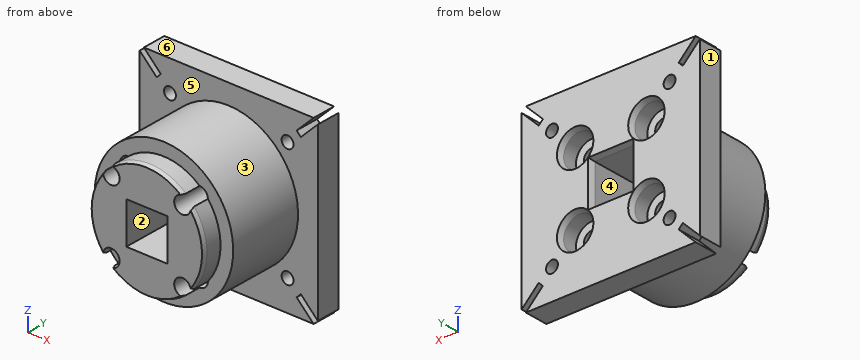
from build123d import *

# Parameters (mm, degrees)
SKETCH1_R           = 17.5
BOSS_EXTRUDE1_DEPTH = 25
SKETCH3_R           = 14.3
BOSS_EXTRUDE2_DEPTH = 5
SKETCH4_W           = 10.4
SKETCH4_H           = 10.4
CUT_EXTRUDE1_DEPTH  = 39.890872965
SKETCH6_R           = 2.1
CUT_EXTRUDE2_DEPTH  = 39.890872965
CHAMFER1_SIZE       = 0.363970234
CHAMFER1_SIZE_2     = 1
SKETCH7_R           = 4.1
CUT_EXTRUDE3_DEPTH  = 5
CHAMFER2_SIZE       = 0.5
CHAMFER2_SIZE2      = 1.37373871
BOSS_EXTRUDE3_START = -6
SKETCH8_W           = 45
SKETCH8_H           = 45
SKETCH8_R           = 17.5
SKETCH8_R_2         = 1.5
BOSS_EXTRUDE3_DEPTH = 6
CUT_EXTRUDE4_DEPTH  = 44.73213928
CHAMFER3_SIZE       = 0.5
CHAMFER3_SIZE2      = 1.37373871


with BuildPart() as part:
    # Sketch1 → Boss-Extrude1 (new body)
    with BuildSketch(Plane(origin=(0, 0, 0), x_dir=(1, 0, 0), z_dir=(0, 1, 0))):
        with Locations(Location((0, 0, 0), (0, 0, 270))):
            Circle(SKETCH1_R)
    extrude(amount=BOSS_EXTRUDE1_DEPTH)

    # Sketch3 → Boss-Extrude2 (add)
    with BuildSketch(Plane.XZ):
        with Locations(Location((0, 0, 0), (0, 0, 90))):
            Circle(SKETCH3_R)
    extrude(amount=BOSS_EXTRUDE2_DEPTH)

    # Sketch4 → Cut-Extrude1 (cut, through all)
    with BuildSketch(Plane(origin=(0, 25, 0), x_dir=(1, 0, 0), z_dir=(0, 1, 0))):
        Rectangle(SKETCH4_W, SKETCH4_H)
    extrude(amount=-CUT_EXTRUDE1_DEPTH, mode=Mode.SUBTRACT)

    # Sketch6 → Cut-Extrude2 (cut, through all)
    with BuildSketch(Plane(origin=(0, 25, 0), x_dir=(1, 0, 0), z_dir=(0, 1, 0))):
        with Locations(Location((9, -9, 0), (0, 0, 270))):
            Circle(SKETCH6_R)
        with Locations(Location((-9, -9, 0), (0, 0, 270))):
            Circle(SKETCH6_R)
        with Locations(Location((-9, 9, 0), (0, 0, 270))):
            Circle(SKETCH6_R)
        with Locations(Location((9, 9, 0), (0, 0, 270))):
            Circle(SKETCH6_R)
    extrude(amount=-CUT_EXTRUDE2_DEPTH, mode=Mode.SUBTRACT)

    # Chamfer1
    # the kernel refuses this chamfer: 1, 0.363970234 mm, written as the material it takes off along each edge
    with BuildSketch(Plane(origin=(0, -5, 0), x_dir=(-0.7601968687413804, 0, 0.649692789521171), z_dir=(-0.649692789521171, 0, -0.7601968687413804))) as chamfer1_piece_1:
        Polygon((14.3 - CHAMFER1_SIZE, 0), (14.3, CHAMFER1_SIZE_2), (14.3, 0), align=None)
    revolve(axis=Axis((0, -5, 0), (0, 1, 0)), revolution_arc=98.963112953, mode=Mode.SUBTRACT)
    with BuildSketch(Plane(origin=(0, -5, 0), x_dir=(-0.6496927895211715, 0, 0.7601968687413799), z_dir=(0.7601968687413799, 0, 0.6496927895211715))) as chamfer1_piece_2:
        Polygon((14.3 - CHAMFER1_SIZE, 0), (14.3, -CHAMFER1_SIZE_2), (14.3, 0), align=None)
    revolve(axis=Axis((0, -5, 0), (0, -1, 0)), revolution_arc=98.963112953, mode=Mode.SUBTRACT)
    with BuildSketch(Plane(origin=(0, -5, 0), x_dir=(-0.7601968687413795, 0, -0.6496927895211719), z_dir=(-0.6496927895211719, 0, 0.7601968687413795))) as chamfer1_piece_3:
        Polygon((14.3, -CHAMFER1_SIZE_2), (14.3 - CHAMFER1_SIZE, 0), (14.3, 0), align=None)
    revolve(axis=Axis((0, -5, 0), (0, -1, 0)), revolution_arc=98.963112953, mode=Mode.SUBTRACT)
    with BuildSketch(Plane(origin=(0, -5, 0), x_dir=(0.6496927895211716, 0, -0.7601968687413798), z_dir=(-0.7601968687413798, 0, -0.6496927895211716))) as chamfer1_piece_4:
        Polygon((14.3, -CHAMFER1_SIZE_2), (14.3 - CHAMFER1_SIZE, 0), (14.3, 0), align=None)
    revolve(axis=Axis((0, -5, 0), (0, -1, 0)), revolution_arc=98.963112953, mode=Mode.SUBTRACT)

    # Sketch7 → Cut-Extrude3 (cut)
    with BuildSketch(Plane(origin=(0, 25, 0), x_dir=(1, 0, 0), z_dir=(0, 1, 0))):
        with Locations(Location((9, 9, 0), (0, 0, 270))):
            Circle(SKETCH7_R)
        with Locations(Location((-9, 9, 0), (0, 0, 270))):
            Circle(SKETCH7_R)
        with Locations(Location((-9, -9, 0), (0, 0, 270))):
            Circle(SKETCH7_R)
        with Locations(Location((9, -9, 0), (0, 0, 270))):
            Circle(SKETCH7_R)
    extrude(amount=-CUT_EXTRUDE3_DEPTH, mode=Mode.SUBTRACT)

    # Chamfer2
    chamfer2_edges = [part.edges().sort_by_distance(p)[0] for p in [
        (5.2, 25, 0),
        (0, 25, -5.2),
        (-5.2, 25, 0),
        (0, 25, 5.2),
    ]]
    chamfer2_side = [part.faces().sort_by_distance(p)[0] for p in [
        (0, 25, -17.005025253),
    ]]
    chamfer(chamfer2_edges, length=CHAMFER2_SIZE, length2=CHAMFER2_SIZE2, reference=chamfer2_side[0])

    # Sketch8 → Boss-Extrude3 (add)
    with BuildSketch(Plane(origin=(0, 25, 0), x_dir=(1, 0, 0), z_dir=(0, 1, 0)).offset(BOSS_EXTRUDE3_START)):
        Rectangle(SKETCH8_W, SKETCH8_H)
        with Locations(Location((0, 0, 0), (0, 0, 270))):
            Circle(SKETCH8_R, mode=Mode.SUBTRACT)
        with Locations(Location((-14.849242405, -14.849242405, 0), (0, 0, 270))):
            Circle(SKETCH8_R_2, mode=Mode.SUBTRACT)
        with Locations(Location((-14.849242405, 14.849242405, 0), (0, 0, 270))):
            Circle(SKETCH8_R_2, mode=Mode.SUBTRACT)
        with Locations(Location((14.849242405, 14.849242405, 0), (0, 0, 270))):
            Circle(SKETCH8_R_2, mode=Mode.SUBTRACT)
        with Locations(Location((14.849242405, -14.849242405, 0), (0, 0, 270))):
            Circle(SKETCH8_R_2, mode=Mode.SUBTRACT)
    extrude(amount=BOSS_EXTRUDE3_DEPTH)

    # Sketch10 → Cut-Extrude4 (cut, through all)
    with BuildSketch(Plane(origin=(0, 25, 0), x_dir=(1, 0, 0), z_dir=(0, 1, 0))):
        Polygon((-18.207999616, -17.147339444), (-17.147339444, -18.207999616), (-21.439339828, -22.5), (-22.5, -22.5), (-22.5, -21.439339828), align=None)
        Polygon((-22.5, 21.439339828), (-18.207999616, 17.147339444), (-17.147339444, 18.207999616), (-21.439339828, 22.5), (-22.5, 22.5), align=None)
        Polygon((21.439339828, 22.5), (17.147339444, 18.207999616), (18.207999616, 17.147339444), (22.5, 21.439339828), (22.5, 22.5), align=None)
        Polygon((17.147339444, -18.207999616), (18.207999616, -17.147339444), (22.5, -21.439339828), (22.5, -22.5), (21.439339828, -22.5), align=None)
    extrude(amount=-CUT_EXTRUDE4_DEPTH, mode=Mode.SUBTRACT)

    # Chamfer3
    chamfer3_edges = [part.edges().sort_by_distance(p)[0] for p in [
        (-9, 25, -13.1),
        (-9, 25, 4.9),
        (9, 25, 4.9),
        (9, 25, -13.1),
    ]]
    chamfer3_side = [part.faces().sort_by_distance(p)[0] for p in [
        (18.843339636, 25, -20.803999808),
    ]]
    chamfer(chamfer3_edges, length=CHAMFER3_SIZE, length2=CHAMFER3_SIZE2, reference=chamfer3_side[0])


solid = part.part
Input: part model. Units: mm. Frame: model coordinates. Face numbers are marked on the shaded views. A direction names the side the tool comes from. Give positions to 0.01 mm unless a question says otherwise; leave off trailing zeros. Order: outer loops, then holes, each group sorted by start corner. A loop starts at its lowest first (then second) coordinate and runs counter-clockwise, first axis right, second up. Notation, with made-up numbers: (-38, -30.75) - (14, -30.75) arc R29 ccw to (14, 0.25) - close; hole circle Ø9 at (18.5, 57.25). An arc over 180 degrees is marked (long way). Write each question's results on one line, items separated by ' | '.
Item 1: Access query for the marked faces 1, 2 and 3. Directions: +Z, -Z, +X, -X, +Y, -Y. A direction counts if a zero-diameter tool reaches every point of the face in a straight line with its end or side. Return the directions, or none.
A:
face 1: +Z, -Z, -X, +Y, -Y | face 2: +Y, -Y | face 3: -Y
Item 2: Material intervals for line 1 along X through (y, z) = (1.5, 0); line 2 along X through (y, z) = (19.5, -2); line 3 along X through (y, z) = (21, -9), sorted ascending.
A:
line 1: x = -17.5 to -5.2, 5.2 to 17.5 | line 2: x = -22.5 to -5.2, 5.2 to 22.5 | line 3: x = -22.5 to -13.1, -4.9 to 4.9, 13.1 to 22.5
Item 3: Section C-C (y = 9.5). Return loops of the section in (x, z).
A:
outline: circle Ø35 at (0, 0); hole circle Ø4.2 at (-9, -9); hole circle Ø4.2 at (-9, 9); hole (-5.2, -5.2) - (5.2, -5.2) - (5.2, 5.2) - (-5.2, 5.2) - close; hole circle Ø4.2 at (9, -9); hole circle Ø4.2 at (9, 9)
Item 4: Section D-D (z = -15). Return loops of the section in (x, y).
A:
outline: (-22.5, 19) - (-16.34, 19) - (-16.34, 25) - (-22.5, 25) - close; (-13.36, 19) - (-9.01, 19) - (-9.01, 0) - (9.01, 0) - (9.01, 19) - (13.36, 19) - (13.36, 25) - (-13.36, 25) - close; (16.34, 19) - (22.5, 19) - (22.5, 25) - (16.34, 25) - close
Item 5: Draft query along Z for the marked faces 4, 5 and 6. Return one class per face: released by +Z, released by -Z, zero draft, split by the parting line, or undercut.
A:
face 4: undercut | face 5: zero draft | face 6: released by +Z
Item 6: Section A-A (x = 0). Return loops of the section in (y, z), and give its area (3 significant figures).
A:
outline: (-5, -13.94) - (-4, -14.3) - (0, -14.3) - (0, -17.5) - (19, -17.5) - (19, -22.5) - (25, -22.5) - (25, -5.7) - (23.63, -5.2) - (-5, -5.2) - close; (-5, 5.2) - (23.63, 5.2) - (25, 5.7) - (25, 22.5) - (19, 22.5) - (19, 17.5) - (0, 17.5) - (0, 14.3) - (-4, 14.3) - (-5, 13.94) - close | area: 765 mm^2
Item 7: Section B-B (z = 0). Return loops of the section in (x, y), and give its area (3 significant figures).
A:
outline: (-22.5, 19) - (-17.5, 19) - (-17.5, 0) - (-14.3, 0) - (-14.3, -4) - (-13.94, -5) - (-5.2, -5) - (-5.2, 23.63) - (-5.7, 25) - (-22.5, 25) - close; (5.2, -5) - (13.94, -5) - (14.3, -4) - (14.3, 0) - (17.5, 0) - (17.5, 19) - (22.5, 19) - (22.5, 25) - (5.7, 25) - (5.2, 23.63) - close | area: 765 mm^2
Item 8: Contact query for flat-ended pins moving along their axis: pin 1 Ø1 at (x, y) = (-3, 3.5) entering from +Z; pin 2 Ø2.5 at (x, z) = (-7, 10) entering from +Y; pin 3 Ø4 at (x, y) = (4, 7.5) entering from +Z. Output: stop coordinate, or through.
A:
pin 1: stops at z = 17.32 | pin 2: stops at y = 20 | pin 3: stops at z = 17.39
